from build123d import *

# Parameters (mm, degrees)
SKETCH1_W                   = 120
SKETCH1_H                   = 80
BOSS_EXTRUDE1_DEPTH         = 10
SKETCH2_R                   = 40
SKETCH2_R_2                 = 30
BOSS_EXTRUDE2_DEPTH         = 20
SKETCH3_R                   = 15
CUT_EXTRUDE1_DEPTH          = 20
SKETCH4_W                   = 20
SKETCH4_H                   = 80
BOSS_EXTRUDE3_DEPTH         = 80
FILLET1_RADIUS              = 40
FILLET1_LENGTH              = 20
SKETCH5_R                   = 16
CUT_EXTRUDE3_DEPTH          = 150.666295471
FILLET1_OF_MIRROR5_2_RADIUS = 40
FILLET1_OF_MIRROR5_2_LENGTH = 20


with BuildPart() as part:
    # Sketch1 → Boss-Extrude1 (new body)
    with BuildSketch(Plane(origin=(0, 0, 0), x_dir=(1, 0, 0), z_dir=(0, 1, 0))):
        Rectangle(SKETCH1_W, SKETCH1_H)
    extrude(amount=BOSS_EXTRUDE1_DEPTH)

    # Sketch2 → Boss-Extrude2 (add)
    with BuildSketch(Plane(origin=(0, 0, 0), x_dir=(1, 0, 0), z_dir=(0, 1, 0))):
        with Locations(Location((0, 0, 0), (0, 0, 270))):
            Circle(SKETCH2_R)
        with Locations(Location((0, 0, 0), (0, 0, 270))):
            Circle(SKETCH2_R_2, mode=Mode.SUBTRACT)
    extrude(amount=BOSS_EXTRUDE2_DEPTH)

    # Sketch3 → Cut-Extrude1 (cut)
    with BuildSketch(Plane(origin=(0, 10, 0), x_dir=(1, 0, 0), z_dir=(0, 1, 0))):
        with Locations(Location((0, -0.840544131, 0), (0, 0, 270))):
            Circle(SKETCH3_R)
    extrude(amount=-CUT_EXTRUDE1_DEPTH, mode=Mode.SUBTRACT)

    # Sketch4 → Boss-Extrude3 (add)
    with BuildSketch(Plane.XZ):
        with Locations((-50, 0)):
            Rectangle(SKETCH4_W, SKETCH4_H)
    boss_extrude3 = extrude(amount=BOSS_EXTRUDE3_DEPTH)

    # Fillet1: full round fillet: the end face becomes a half cylinder, R = half its width
    fillet1_face = Plane((-50, -80, 0), x_dir=(1, 0, 0), z_dir=(0, -1, 0))  # on the end face: x along it, z out of the body
    fillet1_slab = fillet1_face.offset(-FILLET1_RADIUS / 2) * Box(FILLET1_LENGTH, 2 * FILLET1_RADIUS, FILLET1_RADIUS, mode=Mode.PRIVATE)  # the body's end, R deep
    fillet1_round = Plane((-50, -40, 0), x_dir=(0, -1, 0), z_dir=(1, 0, 0)) * Cylinder(FILLET1_RADIUS, FILLET1_LENGTH, mode=Mode.PRIVATE)  # its axis R under the face
    add(fillet1_slab - fillet1_round, mode=Mode.SUBTRACT)

    # Sketch5 → Cut-Extrude3 (cut, through all)
    with BuildSketch(Plane.ZY.offset(60)):
        with Locations((0, -40)):
            Circle(SKETCH5_R)
    cut_extrude3 = extrude(amount=-CUT_EXTRUDE3_DEPTH, mode=Mode.SUBTRACT)

    # Mirror5: Boss-Extrude3 across plane
    add(boss_extrude3.mirror(Plane(origin=(0, 0, 0), x_dir=(0, 0, 1), z_dir=(1, 0, 0))))

    # Fillet1 of Mirror5 2: full round fillet: the end face becomes a half cylinder, R = half its width
    fillet1_of_mirror5_2_face = Plane((50, -80, 0), x_dir=(-1, 0, 0), z_dir=(0, -1, 0))  # on the end face: x along it, z out of the body
    fillet1_of_mirror5_2_slab = fillet1_of_mirror5_2_face.offset(-FILLET1_OF_MIRROR5_2_RADIUS / 2) * Box(FILLET1_OF_MIRROR5_2_LENGTH, 2 * FILLET1_OF_MIRROR5_2_RADIUS, FILLET1_OF_MIRROR5_2_RADIUS, mode=Mode.PRIVATE)  # the body's end, R deep
    fillet1_of_mirror5_2_round = Plane((50, -40, 0), x_dir=(0, -1, 0), z_dir=(-1, 0, 0)) * Cylinder(FILLET1_OF_MIRROR5_2_RADIUS, FILLET1_OF_MIRROR5_2_LENGTH, mode=Mode.PRIVATE)  # its axis R under the face
    add(fillet1_of_mirror5_2_slab - fillet1_of_mirror5_2_round, mode=Mode.SUBTRACT)

    # Mirror6: Cut-Extrude3 across plane
    add(cut_extrude3.mirror(Plane(origin=(0, 0, 0), x_dir=(0, 0, 1), z_dir=(1, 0, 0))), mode=Mode.SUBTRACT)


solid = part.part
Input: part model. Units: mm. Frame: model coordinates. A direction names the side the tool comes from. Round coordinates to 2 decimals unless told otherwise and drop trailing zeros. Order: outer loops, then holes, each group sorted by start corner. A loop starts at its lowest first (then second) coordinate and runs counter-clockwise, first axis right, second up. Notation, with made-up numbers: (29, 35) - (70, 35) arc R17 cw to (70, 55) - close; hole circle Ø11 at (-39.5, -24). An arc over 180 degrees is marked (long way). Use a Markdown table: item, result.
1. First-contact query: pin 1 (5 mm diameter, centred on x = -32, z = 29, fed in from -Y); pin 2 (10 mm diameter, centred on x = 5.5, z = 17, fed in from +Y). Flat tips, straight axial feed; report the tip coordinate or a pass-through.
Evaluation:
| item | result |
|---|---|
| pin 1 | y = 0 |
| pin 2 | y = 10 |
2. Section A-A on y = -6. Return the cut outline in (x, z), then the cut area to 3 significant figures.
Evaluation:
| item | result |
|---|---|
| outline | (-60, -40) - (-40, -40) - (-40, 40) - (-60, 40) - close; (40, -40) - (60, -40) - (60, 40) - (40, 40) - close |
| area | 3,200 mm^2 |
3. Section D-D on x = 12. Return the cut outline in (y, z).
Evaluation:
| item | result |
|---|---|
| outline | (0, -40) - (10, -40) - (10, -38.16) - (20, -38.16) - (20, -27.5) - (10, -27.5) - (10, -8.16) - (0, -8.16) - close; (0, 9.84) - (10, 9.84) - (10, 27.5) - (20, 27.5) - (20, 38.16) - (10, 38.16) - (10, 40) - (0, 40) - close |
4. Material intervals for probe 1 along X at (y, z) = (-9, -34.5); probe 2 along Y at (x, z) = (-46.5, 0); probe 3 along X at (y, z) = (16.25, 0), sorted ascending.
Evaluation:
| item | result |
|---|---|
| probe 1 | -60 to -40, 40 to 60 |
| probe 2 | -80 to -56, -24 to 10 |
| probe 3 | -40 to -30, 30 to 40 |
5. Section B-B on x = 52.5. Return the cut outline in (y, z), then the cut area to 3 significant figures.
Evaluation:
| item | result |
|---|---|
| outline | (-40, -40) - (10, -40) - (10, 40) - (-40, 40) arc R40 ccw to start; hole circle Ø32 at (-40, 0) |
| area | 5,710 mm^2 |
6. Mould query, pull axis Z, two halves, no side actions, for faces 6 (the face through (-50.14, -55.62, -3.47)), 7 (the face through (-49.86, -79.99, 0.88)), 8 (the face through (-60, -24, -9)), 9 (the face through (0.66, 5.07, -14.145)). Classes: +Z half, -Z half, draft (parallel to the pull), parting line (faces both ways), or undercut.
Evaluation:
| item | result |
|---|---|
| face 6 | undercut |
| face 7 | parting line |
| face 8 | draft |
| face 9 | undercut |
7. Access query for faces 1 (the face through (-44, 10, -1)), 2 (the face through (17, 0, -1)), 3 (the face through (13, 10, -7)), 4 (the face through (14, 2, -40)), 5 (the face through (43, 10, -1)). Directions: +Z, -Z, +X, -X, +Y, -Y. A direction counts if a zero-diameter tool reaches every point of the face in a straight line with its end or side. Return the directions, or none.
Evaluation:
| item | result |
|---|---|
| face 1 | -X, +Y |
| face 2 | +Z, -Z, -Y |
| face 3 | +Y |
| face 4 | -Z, +X, -X, +Y, -Y |
| face 5 | +X, +Y |
8. Section C-C on z = 0. Return the cut outline in (x, y), then the cut area to 3 significant figures.
Evaluation:
| item | result |
|---|---|
| outline | (-60, -80) - (-40, -80) - (-40, -56) - (-60, -56) - close; (-60, -24) - (-40, -24) - (-40, 0) - (-14.98, 0) - (-14.98, 10) - (-30, 10) - (-30, 20) - (-40, 20) - (-40, 10) - (-60, 10) - close; (14.98, 0) - (40, 0) - (40, -24) - (60, -24) - (60, 10) - (40, 10) - (40, 20) - (30, 20) - (30, 10) - (14.98, 10) - close; (40, -80) - (60, -80) - (60, -56) - (40, -56) - close |
| area | 3,020 mm^2 |
